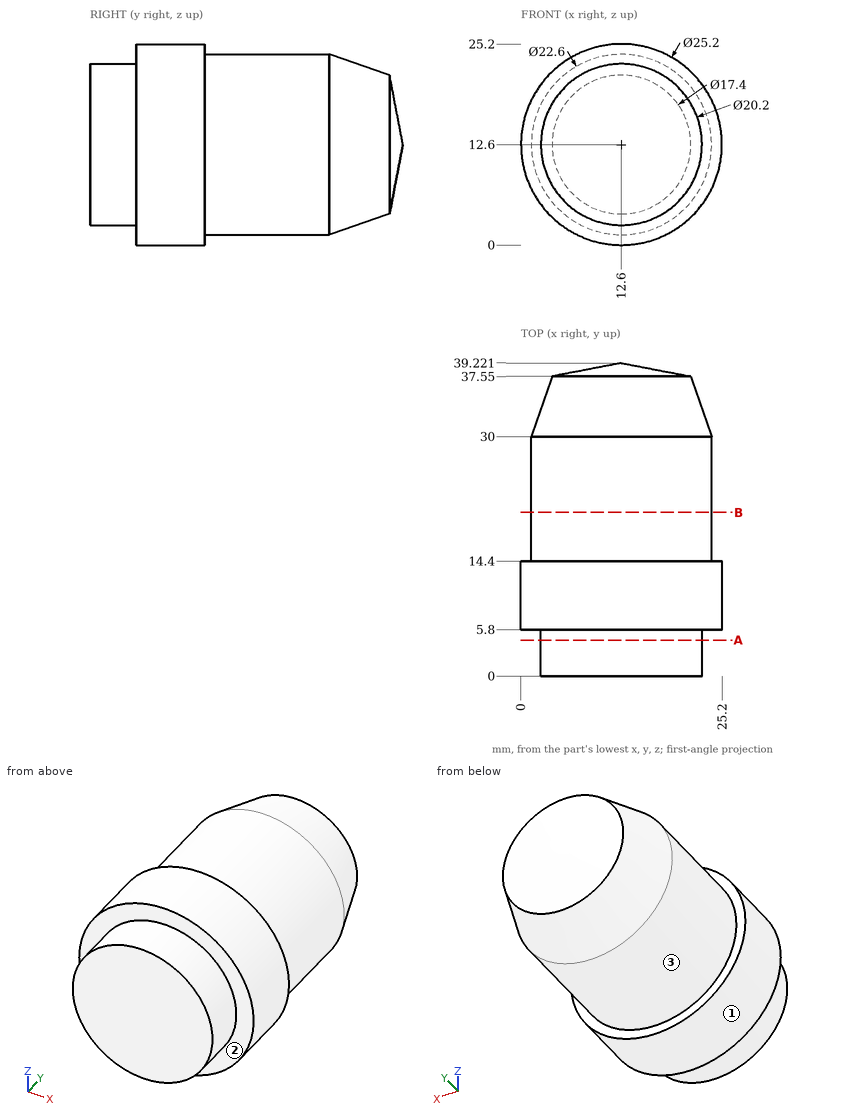
The figure shows three views and two pictorial views of one solid part (mm, origin at its lowest corner). Answer the questions. A direction names the side the tool comes from. Give positions to 0.01 mm unless a question says otherwise; leave off trailing zeros. Write each loop counter-clockwise with the first axis right and the second up, starting at its lowest first coordinate (ties: lowest second). Pieces come first, ordered by that corner, then holes. Notation, with made-up numbers: (61.5, 2) - (102.5, 2) arc R17 cw to (102.5, 11) - close; hole circle Ø8 at (32.25, 46). An arc over 180 degrees is marked (long way). Use one line per item in the form item = value. Start each with the question number.
1) Consider line 1 along Z through (x, y) = (15.5, 11); line 2 along Z through (x, y) = (9.5, 4); line 3 along X through (y, z) = (35.5, 8.75). Determine where each line is inside the solid, lowest interval first. Write a range as from..to.
2) Flat-ended cylindrical pins translate along their axes: pin 1 Ø2 at (x, y) = (17.5, 31.5) entering from +Z; pin 2 Ø5 at (x, y) = (19, 13) entering from -Z; pin 3 Ø5 at (y, z) = (34, 6) entering from -X. Find the tip coordinate at first contact, or state that the pin passes through.
3) Find section A-A on y = 4.5. Determine the outline of the cut face in (x, z).
4) Find section B-B on y = 20.5. Determine the outline of the cut face in (x, z), plus the area to 3 significant figures.
5) A tool of negligible diameter and unlimited length cuts with its end or side. For the marked faces 1, 2 and 3, from which of +Z, -Z, +X, -X, +Y, -Y can it reach the whole face along a straight path? Write none if from no direction.
Geometry results:
q1.line_1 = 0.34..24.86
q1.line_2 = 2.99..22.21
q1.line_3 = 4.02..21.18
q2.pin_1 = 22.8
q2.pin_2 = 0.62
q2.pin_3 = 3.23
q3.outline = circle Ø20.2 at (12.6, 12.6)
q4.outline = circle Ø22.6 at (12.6, 12.6)
q4.area = 401 mm2
q5.face_1 = +Y, -Y
q5.face_2 = -Y
q5.face_3 = +Y
